Geometry check sheet. Reference: the model listing, model coordinates, mm. Face numbers are marked on the shaded views. A direction names the side the tool comes from. Coordinates: 2 decimals unless noted, no trailing zeros. Write each loop counter-clockwise with the first axis right and the second up, starting at its lowest first coordinate (ties: lowest second). Pieces come first, ordered by that corner, then holes. Notation, with made-up numbers: (70, -35) -> (99, -35) arc R28 cw to (99, -2) -> close; hole circle Ø2 at (87, 43). An arc over 180 degrees is marked (long way). Answer in a Markdown table with one row per item. Add a question column.
Q1. Thickness scan on line 1 (Y direction, x = 0, z = 6.9); line 2 (Y direction, x = 0, z = 6); line 3 (Y direction, x = -1.25, z = 2.75). Record the ranges inside material, lowest first.
Q2. Section check D-D, the plane x = -2. Record the boundary of the cut face in (y, z), and give its area (3 significant figures).
Q3. Tool access check on the marked faces 4 and 5. Record the directions out of +Z, -Z, +X, -X, +Y, -Y that give a thin tool (end or side, any length) a straight path to the whole face; none if there is none.
Q4. Section check C-C, the plane z = 2.5. Record the boundary of the cut face in (x, y) (1 decimal), and give its area (3 significant figures).
Q5. Gauge pin test, flat ends, axial feed: P1, Ø5, axis at y = 1, z = 1, coming from the -X side; P2, Ø4, axis at x = -3.5, z = 5.5, coming from the +Y side; P3, Ø4.5, axis at x = -1.5, y = 8.5, coming from the -Z side; P4, Ø2, axis at x = -3, z = 5.5, coming from the -Y side. Record the tip position at first contact, or that the pin passes through.
Q6. Release check for a two-part mould opening along X. For the marked faces 1, 2 and 3 record: pulls with the +X half, pulls with the -X half, needs draft (parallel to the pull), parting line crosses it, or undercut.
Q7. Section check B-B, the plane y = -0.25. Record the boundary of the cut face in (x, z).
Q8. Section check A-A, the plane x = 0. Record the boundary of the cut face in (y, z).
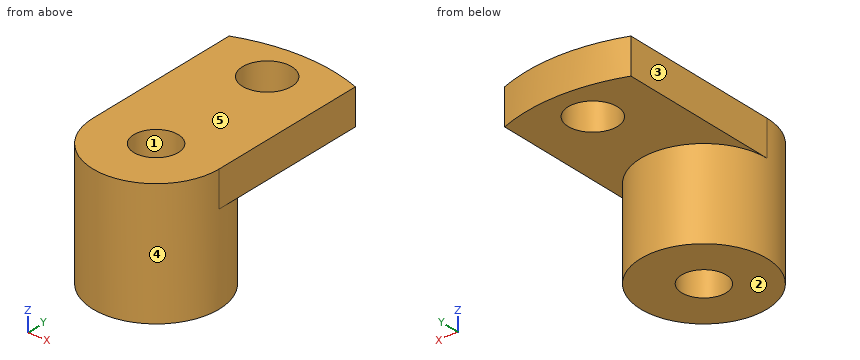
```python
from build123d import *

# Parameters (mm, degrees)
F0_R     = 4.4958
F0_R_2   = 1.5875
F1_DEPTH = 6.35
F2_R     = 12.7
F2_R_2   = 1.7526
F2_R_3   = 1.5875
F3_DEPTH = 2.54
F4_W     = 58.600948
F4_H     = 48.189808
F5_DEPTH = 25.4


with BuildPart() as f1:
    # F0 (on Top) → F1 (new body)
    with BuildSketch(Plane.XY):
        Circle(F0_R)
        Circle(F0_R_2, mode=Mode.SUBTRACT)
    extrude(amount=F1_DEPTH)

    # F2 (on face) → F3 (join)
    with BuildSketch(Plane.XY.offset(6.35)):
        Circle(F2_R)
        with Locations((0, -9.6901)):
            Circle(F2_R_2, mode=Mode.SUBTRACT)
        with Locations((-8.391873, -4.84505)):
            Circle(F2_R_2, mode=Mode.SUBTRACT)
        Circle(F2_R_3, mode=Mode.SUBTRACT)
        with Locations((8.391873, -4.84505)):
            Circle(F2_R_2, mode=Mode.SUBTRACT)
        with Locations((-8.391873, 4.84505)):
            Circle(F2_R_2, mode=Mode.SUBTRACT)
        with Locations((0, 9.6901)):
            Circle(F2_R_2, mode=Mode.SUBTRACT)
        with Locations((8.391873, 4.84505)):
            Circle(F2_R_2, mode=Mode.SUBTRACT)
    extrude(amount=F3_DEPTH)

    # F4 (on face) → F5 (cut)
    with BuildSketch(Plane.XY.offset(8.89)):
        Rectangle(F4_W, F4_H)
        with BuildLine():
            ThreePointArc((4.4958, 0), (0, -4.4958), (-4.4958, 0))
            Line((-4.4958, 0), (-4.4958, 11.877617))
            ThreePointArc((-4.4958, 11.877617), (0, 12.7), (4.4958, 11.877617))
            Line((4.4958, 11.877617), (4.4958, 0))
        make_face(mode=Mode.SUBTRACT)
    extrude(amount=-F5_DEPTH, mode=Mode.SUBTRACT)


solid = f1.part
```
Calculated:
| question | item | result |
|---|---|---|
| 1 | line 1 | y = -4.5 to -1.59, 1.59 to 7.94, 11.44 to 12.7 |
| 1 | line 2 | y = -4.5 to -1.59, 1.59 to 4.5 |
| 1 | line 3 | y = -4.32 to -0.98, 0.98 to 4.32 |
| 2 | outline | (-4.03, 0) -> (4.03, 0) -> (4.03, 6.35) -> (12.54, 6.35) -> (12.54, 8.89) -> (-4.03, 8.89) -> close |
| 2 | area | 93.2 mm² |
| 3 | face 4 | -Z |
| 3 | face 5 | +Z, +X, -X, +Y, -Y |
| 4 | outline | circle Ø9 at (0, 0); hole circle Ø3.2 at (0, 0) |
| 4 | area | 55.6 mm² |
| 5 | P1 | stops at x = -4.5 |
| 5 | P2 | stops at y = 12.59 |
| 5 | P3 | stops at z = 6.35 |
| 5 | P4 | stops at y = -4.03 |
| 6 | face 1 | undercut |
| 6 | face 2 | needs draft |
| 6 | face 3 | pulls with the -X half |
| 7 | outline | (-4.49, 0) -> (-1.57, 0) -> (-1.57, 8.89) -> (-4.49, 8.89) -> close; (1.57, 0) -> (4.49, 0) -> (4.49, 8.89) -> (1.57, 8.89) -> close |
| 8 | outline | (-4.5, 0) -> (-1.59, 0) -> (-1.59, 8.89) -> (-4.5, 8.89) -> close; (1.59, 0) -> (4.5, 0) -> (4.5, 6.35) -> (7.94, 6.35) -> (7.94, 8.89) -> (1.59, 8.89) -> close; (11.44, 6.35) -> (12.7, 6.35) -> (12.7, 8.89) -> (11.44, 8.89) -> close |
